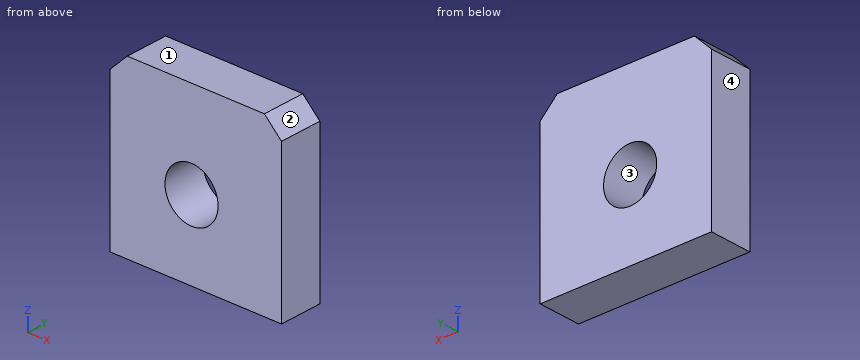
```python
from build123d import *

# Parameters (mm, degrees)
SKETCH_1_W          = 20
SKETCH_1_H          = 20
EXTRUDE_1_DEPTH     = 5
SKETCH_2_R          = 3.1
CUT_EXTRUDE_1_DEPTH = 5
CHAMFER_1_SIZE      = 2


with BuildPart() as part:
    # 스케치1 → 보스-돌출1 (new body)
    with BuildSketch(Plane(origin=(0, 0, 0), x_dir=(1, 0, 0), z_dir=(0, 1, 0))):
        with Locations((10, 10)):
            Rectangle(SKETCH_1_W, SKETCH_1_H)
    extrude(amount=EXTRUDE_1_DEPTH)

    # 스케치2 → 컷-돌출1 (cut)
    with BuildSketch(Plane(origin=(0, 5, 0), x_dir=(1, 0, 0), z_dir=(0, 1, 0))):
        with Locations(Location((9.5, 11, 0), (0, 0, 270))):
            Circle(SKETCH_2_R)
    extrude(amount=-CUT_EXTRUDE_1_DEPTH, mode=Mode.SUBTRACT)

    # 모따기1
    chamfer_1_edges = [part.edges().sort_by_distance(p)[0] for p in [
        (20, 2.5, 0),
        (0, 2.5, 0),
    ]]
    chamfer(chamfer_1_edges, length=CHAMFER_1_SIZE)


solid = part.part
```
Could you check a few things on this model? Use its own coordinates, in mm. Face numbers are marked on the shaded views. Coordinates: 2 decimals unless noted, no trailing zeros. Write each loop counter-clockwise with the first axis right and the second up, starting at its lowest first coordinate (ties: lowest second). Pieces come first, ordered by that corner, then holes. Notation, with made-up numbers: (40, 23) -> (86, 23) arc R30 ccw to (86, 45) -> close; hole circle Ø4 at (47, 32.25). An arc over 180 degrees is marked (long way). Return JSON: item names as keys, results as strings.
(1) We'd pull the mould along X, two halves only. Please class the marked faces 1, 2, 3 and 4: +X half, -X half, draft (parallel to the pull), parting line (faces both ways), or undercut.
Numbers:
{"face 1": "draft", "face 2": "+X half", "face 3": "undercut", "face 4": "-X half"}
(2) Imagine slicing it at C-C, the plane x = 9.5. Please give me the cut outline in (y, z), then the cut area to 3 significant figures.
Numbers:
{"outline": "(0, -20) -> (5, -20) -> (5, -14.1) -> (0, -14.1) -> close; (0, -7.9) -> (5, -7.9) -> (5, 0) -> (0, 0) -> close", "area": "69.0 mm2"}
(3) Imagine slicing it at A-A, the plane y = 0.45. Please give me the cut outline in (x, z).
Numbers:
{"outline": "(0, -20) -> (20, -20) -> (20, -2) -> (18, 0) -> (2, 0) -> (0, -2) -> close; hole circle Ø6.2 at (9.5, -11)"}
(4) Imagine slicing it at D-D, the plane x = 18.75. Please give me the cut outline in (y, z).
Numbers:
{"outline": "(0, -20) -> (5, -20) -> (5, -0.75) -> (0, -0.75) -> close"}
(5) I need wall thicknesses on L1, parallel to X at y = 1.5, z = -11; L2, parallel to X at y = 4.25, z = -11.75; L3, parallel to Z at x = 18.75, y = 2.35. Which ranges of each line are inside material? Lowest first, please.
Numbers:
{"L1": "x = 0 to 6.4, 12.6 to 20", "L2": "x = 0 to 6.49, 12.51 to 20", "L3": "z = -20 to -0.75"}
(6) Imagine slicing it at B-B, the plane z = -11. Please give me the cut outline in (x, y).
Numbers:
{"outline": "(0, 0) -> (6.4, 0) -> (6.4, 5) -> (0, 5) -> close; (12.6, 0) -> (20, 0) -> (20, 5) -> (12.6, 5) -> close"}
